Can you work these out from the model? Positions are in its coordinate system, mm. A direction names the side the tool comes from. Round coordinates to 2 decimals unless told otherwise and drop trailing zeros. Write each loop counter-clockwise with the first axis right and the second up, starting at its lowest first coordinate (ties: lowest second). Pieces come first, ordered by that corner, then holes. Notation, with made-up numbers: M 19,12.5 L 63,12.5 A9 ccw 63,27.5 Z; hole C 81,33.25 d8. An arc over 180 degrees is marked long. Answer in a Markdown table with one row per item. Add a question column.
(1) Suppose I cut it at B-B, the plane y = 8.5. Count the separate pieces of the cut face and the enclosed holes in it, then the cut area to 3 significant figures.
(2) If I drill on probe 1 along X at (y, z) = (11.5, 0); probe 2 along X at (y, z) = (7.25, -1); probe 3 along X at (y, z) = (11, 3.75), over which ranges is the centre line in solid material (lowest first)?
(3) Suppose I cut it at D-D, the plane z = 5.5. Write out the boundary of the cut face in (x, y), then the cut area to 3 significant figures.
(4) If we mould it in two halves opening along X, with no side actions, what happens to faces 1 (the face through (25.4, 9, 0)), 2 (the face through (-25.4, 9, 0)), 3 (the face through (0, 19.05, -4)), 4 (the face through (-16, 3.175, 0))? For each: released by +X, released by -X, zero draft, split by the parting line, or undercut.
(5) Suppose I cut it at C-C, the plane x = -3. Write out the boundary of the cut face in (y, z) (3 decimals), then the cut area to 3 significant figures.
(6) For faces 5 (the face through (7.938, 10, 2)), 6 (the face through (19.023, 11.224, -0.413)), 7 (the face through (17, 9, 6.35)), which set-ups out of +Z, -Z, +X, -X, +Y, -Y let a thin tool reach every point of the face, with its end or its side?
(7) I'm going to push flat-ended pins straight in: pin 1 (2 mm diameter, centred on x = -1.5, y = 17, fed in from +Z) (3 decimals); pin 2 (3 mm diameter, centred on x = 14.5, z = 0.5, fed in from +Y) (3 decimals). Where does each tip first touch, or does it pass through?
from build123d import *

# Parameters (mm, degrees)
SKETCH1_W           = 50.8
SKETCH1_H           = 12.7
BOSS_EXTRUDE1_DEPTH = 19.05
SKETCH2_R           = 3.175
CUT_EXTRUDE1_DEPTH  = 15.875
SKETCH3_W           = 15.875
SKETCH3_H           = 9.525
CUT_EXTRUDE2_DEPTH  = 33.378773911


with BuildPart() as part:
    # Sketch1 → Boss-Extrude1 (new body)
    with BuildSketch(Plane(origin=(0, 0, 0), x_dir=(1, 0, 0), z_dir=(0, 1, 0))):
        Rectangle(SKETCH1_W, SKETCH1_H)
    extrude(amount=BOSS_EXTRUDE1_DEPTH)

    # Sketch2 → Cut-Extrude1 (cut)
    with BuildSketch(Plane(origin=(0, 19.05, 0), x_dir=(1, 0, 0), z_dir=(0, 1, 0))):
        with Locations(Location((-15.875, 0, 0), (0, 0, 270))):
            Circle(SKETCH2_R)
        with Locations(Location((15.875, 0, 0), (0, 0, 270))):
            Circle(SKETCH2_R)
    extrude(amount=-CUT_EXTRUDE1_DEPTH, mode=Mode.SUBTRACT)

    # Sketch3 → Cut-Extrude2 (cut, through all)
    with BuildSketch(Plane(origin=(0, 19.05, 0), x_dir=(1, 0, 0), z_dir=(0, 1, 0))):
        with Locations((0, -1.5875)):
            Rectangle(SKETCH3_W, SKETCH3_H)
    extrude(amount=-CUT_EXTRUDE2_DEPTH, mode=Mode.SUBTRACT)


solid = part.part
Calculated:
| question | item | result |
|---|---|---|
| 1 | separate pieces | 1 |
| 1 | enclosed holes | 2 |
| 1 | area | 431 mm² |
| 2 | probe 1 | -25.4 to -19.05, -12.7 to -7.94, 7.94 to 12.7, 19.05 to 25.4 |
| 2 | probe 2 | -25.4 to -18.89, -12.86 to -7.94, 7.94 to 12.86, 18.89 to 25.4 |
| 2 | probe 3 | -25.4 to -7.94, 7.94 to 25.4 |
| 3 | outline | M -25.4,0 L -7.94,0 L -7.94,19.05 L -25.4,19.05 Z; M 7.94,0 L 25.4,0 L 25.4,19.05 L 7.94,19.05 Z |
| 3 | area | 665 mm² |
| 4 | face 1 | released by +X |
| 4 | face 2 | released by -X |
| 4 | face 3 | zero draft |
| 4 | face 4 | undercut |
| 5 | outline | M 0,-6.35 L 19.05,-6.35 L 19.05,-3.175 L 0,-3.175 Z |
| 5 | area | 60.5 mm² |
| 6 | face 5 | +Z, +Y, -Y |
| 6 | face 6 | +Y |
| 6 | face 7 | +Z, +X, -X, +Y, -Y |
| 7 | pin 1 | z = -3.175 |
| 7 | pin 2 | y = 3.175 |
